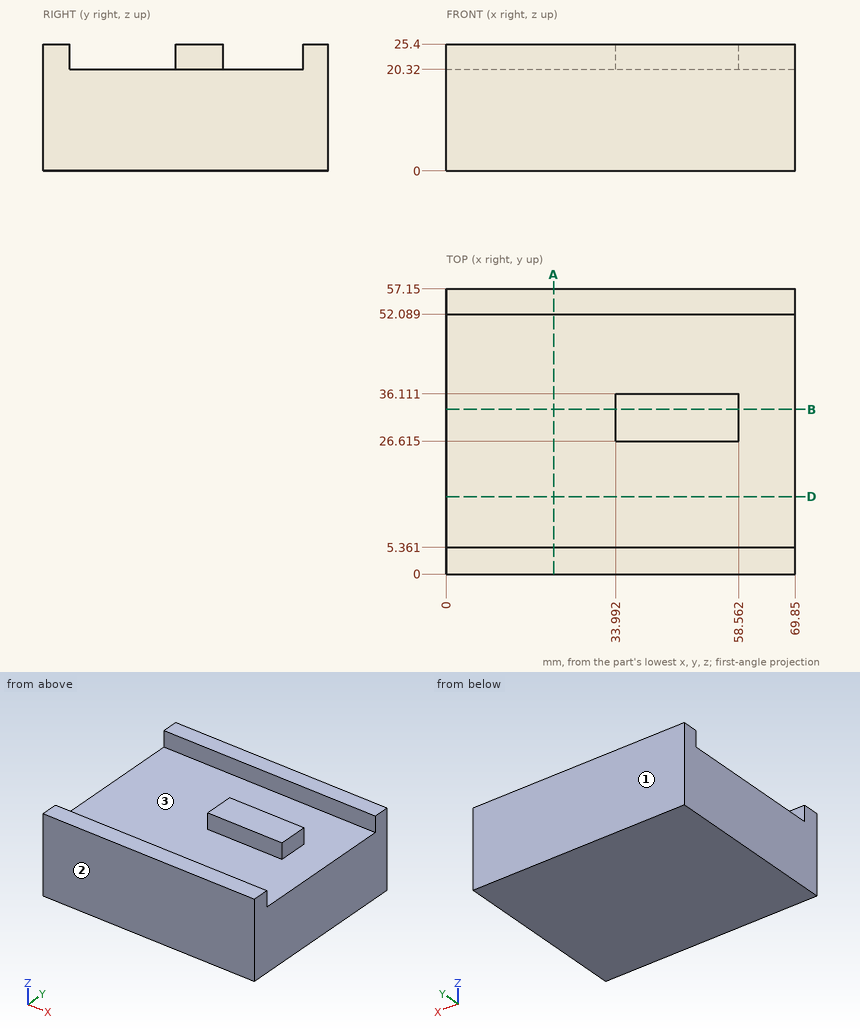
Geometry: see drawing. Coordinates: mm, zero at the bounding-box minimum. Give positions to 0.01 mm unless a question says otherwise; leave off trailing zeros. Loops run counter-clockwise (first coordinate to the right, second up) from the corner with the lowest first, then second, coordinate; pieces in that order, holes last. Notation, with made-up numbers: (87.5, 64.25) - (119.5, 64.25) arc R3 cw to (119.5, 68.25) - close; hole circle Ø11 at (42.25, 52.25). An arc over 180 degrees is marked (long way). Use CSV: the item, a comma, the result in double quotes. Start each with the question number.
Item 1: Section B-B on y = 33. Return loops of the section in (x, z).
Item 2: Section A-A on x = 21.5. Return loops of the section in (y, z).
Item 3: Mould query, pull axis Y, two halves, no side actions, for the marked faces 1, 2 and 3. Classes: pulls with the +Y half, pulls with the -Y half, needs draft (parallel to the pull), parting line crosses it, or undercut.
Item 4: Line query: line 1 (Y direction, x = 64.5, z = 24.5); line 2 (Z direction, x = 30.5, y = 38.5). Output: solid intervals per line, ascending.
Item 5: Section D-D on y = 15.5. Return loops of the section in (x, z).
Item 6: Contact query for flat-ended pins moving along their axis: P1, Ø6, axis at x = 10, y = 28.5, coming from the +Z side; P2, Ø1.5, axis at y = 31.5, z = 22, coming from the +X side; P3, Ø4, axis at y = 31.5, z = 22.5, coming from the -X side. Output: stop coordinate, or through.
Ans:
1,outline,"(0, 0) - (69.85, 0) - (69.85, 20.32) - (58.56, 20.32) - (58.56, 25.4) - (33.99, 25.4) - (33.99, 20.32) - (0, 20.32) - close"
2,outline,"(0, 0) - (57.15, 0) - (57.15, 25.4) - (52.09, 25.4) - (52.09, 20.32) - (5.36, 20.32) - (5.36, 25.4) - (0, 25.4) - close"
3,face 1,"pulls with the +Y half"
3,face 2,"pulls with the -Y half"
3,face 3,"undercut"
4,line 1,"y = 0 to 5.36, 52.09 to 57.15"
4,line 2,"z = 0 to 20.32"
5,outline,"(0, 0) - (69.85, 0) - (69.85, 20.32) - (0, 20.32) - close"
6,P1,"stops at z = 20.32"
6,P2,"stops at x = 58.56"
6,P3,"stops at x = 33.99"
